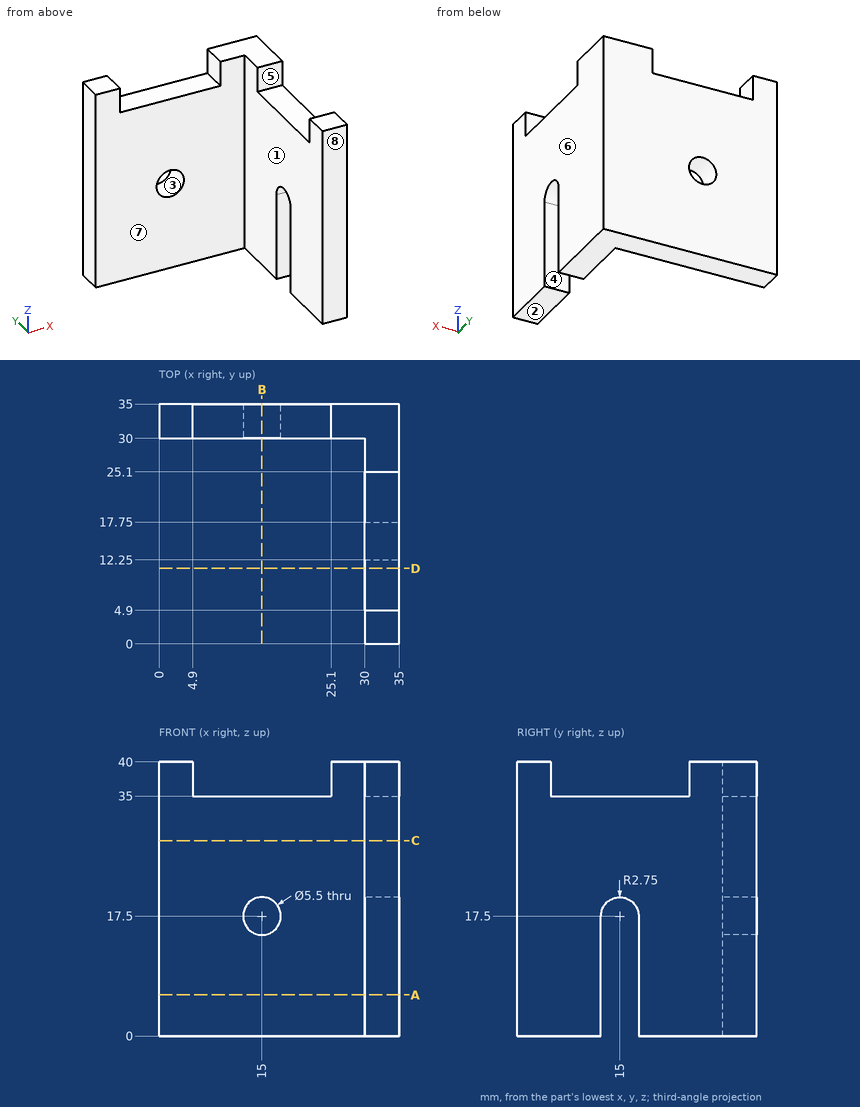
Verification items for this drawing (mm, ordinates from the low corner). A direction names the side the tool comes from. Coordinates: 2 decimals unless noted, no trailing zeros. Loops run counter-clockwise (first coordinate to the right, second up) from the corner with the lowest first, then second, coordinate; pieces in that order, holes last. Notation, with made-up numbers: (-15.5, 89.5) - (40.5, 89.5) arc R6 cw to (40.5, 95.5) - close; hole circle Ø7 at (-22.75, -28.75). An arc over 180 degrees is marked (long way). Use one line per item in the form item = value. Start each with the question number.
Item 1: Section check B-B, the plane x = 15. Enter the section's corners in (y, z).
Item 2: Section check A-A, the plane z = 6. Enter the section's corners in (x, y).
Item 3: Tool access check on the marked faces 4, 5, 6, 7 and 8. Record the directions out of +Z, -Z, +X, -X, +Y, -Y that give a thin tool (end or side, any length) a straight path to the whole face; none if there is none.
Item 4: Thickness scan on probe 1 along Z at (x, y) = (15, 32.05); probe 2 along X at (y, z) = (28.5, 29). Record the ranges inside material, lowest first.
Item 5: Mould release check, pull along Z, two halves, no side actions. Record for the marked faces 1, 2 and 3: +Z half, -Z half, draft (parallel to the pull), parting line (faces both ways), or undercut.
Item 6: Section check D-D, the plane y = 11. Enter the section's corners in (x, z).
Item 7: Section check C-C, the plane z = 28.5. Enter the section's corners in (x, y).
Item 8: Gauge pin test, flat ends, axial feed: pin 1 (1.5 mm diameter, centred on x = 32.5, y = 12, fed in from +Z); pin 2 (2.5 mm diameter, centred on y = 32, z = 37, fed in from -X); pin 3 (6 mm diameter, centred on y = 24, z = 19, fed in from -X); pin 4 (5 mm diameter, centred on x = 15, z = 17.5, fed in from -Y). Record the tip position at first contact, or that the pin passes through.
Computed:
q1.outline = (30, 0) - (35, 0) - (35, 14.75) - (30, 14.75) - close; (30, 20.25) - (35, 20.25) - (35, 35) - (30, 35) - close
q2.outline = (0, 30) - (30, 30) - (30, 17.75) - (35, 17.75) - (35, 35) - (0, 35) - close; (30, 0) - (35, 0) - (35, 12.25) - (30, 12.25) - close
q3.face_4 = -Z, +X, -X
q3.face_5 = +Z, +X, -X
q3.face_6 = +Z, -Z, +X, +Y, -Y
q3.face_7 = +Z, -Z, -X, -Y
q3.face_8 = +Z, -Z, +X, -X, -Y
q4.probe_1 = 0 to 14.75, 20.25 to 35
q4.probe_2 = 30 to 35
q5.face_1 = draft
q5.face_2 = -Z half
q5.face_3 = undercut
q6.outline = (30, 0) - (35, 0) - (35, 35) - (30, 35) - close
q7.outline = (0, 30) - (30, 30) - (30, 0) - (35, 0) - (35, 35) - (0, 35) - close
q8.pin_1 = 35
q8.pin_2 = 0
q8.pin_3 = 30
q8.pin_4 = through
